Input: part model. Units: mm. Frame: model coordinates. Face numbers are marked on the shaded views. A direction names the side the tool comes from. Coordinates: 2 decimals unless noted, no trailing zeros. Write each loop counter-clockwise with the first axis right and the second up, starting at its lowest first coordinate (ties: lowest second). Pieces come first, ordered by that corner, then holes.
from build123d import *

# Parameters (mm, degrees)
SKETCH1_W            = 31.75
SKETCH1_H            = 44.45
BOSS_EXTRUDE1_DEPTH  = 4.7625
SKETCH2_R            = 1.5
SKETCH2_R_2          = 2
CUT_EXTRUDE1_DEPTH   = 5.7625
FILLET1_R            = 2.54
SKETCH3_W            = 27
SKETCH3_H            = 8
CUT_EXTRUDE2_DEPTH   = 5.7625
FILLET2_R            = 1
SKETCH4_R            = 7.9375
SKETCH4_R_2          = 4
BOSS_EXTRUDE2_DEPTH  = 4.7625
SKETCH5_R            = 4
CUT_EXTRUDE3_DEPTH   = 4.7625
SKETCH6_R            = 5.715
CUT_EXTRUDE4_DEPTH   = 3.175
CUT_REVOLVE1_ANGLE   = 90
FILLET3_R            = 5.08
FILLET3_OF_MIRROR1_R = 5.08
BOSS_EXTRUDE3_DEPTH  = 4.7625


with BuildPart() as part:
    # Sketch1 → Boss-Extrude1 (new body)
    with BuildSketch(Plane.XY):
        Rectangle(SKETCH1_W, SKETCH1_H)
    extrude(amount=BOSS_EXTRUDE1_DEPTH)

    # Sketch2 → Cut-Extrude1 (cut, through all)
    with BuildSketch(Plane.XY.offset(4.7625)):
        with Locations((-12.7, 19.05)):
            Circle(SKETCH2_R)
        with Locations((12.7, 19.05)):
            Circle(SKETCH2_R)
        with Locations((0, -17.78)):
            Circle(SKETCH2_R_2)
        with Locations((12.7, -19.05)):
            Circle(SKETCH2_R)
        with Locations((-12.7, -19.05)):
            Circle(SKETCH2_R)
    extrude(amount=-CUT_EXTRUDE1_DEPTH, mode=Mode.SUBTRACT)

    # Fillet1
    fillet1_edges = [part.edges().sort_by_distance(p)[0] for p in [
        (15.875, -22.225, 2.38125),
        (-15.875, -22.225, 2.38125),
        (-15.875, 22.225, 2.38125),
        (15.875, 22.225, 2.38125),
    ]]
    fillet(fillet1_edges, radius=FILLET1_R)

    # Sketch3 → Cut-Extrude2 (cut, through all)
    with BuildSketch(Plane.XY.offset(4.7625)):
        with Locations((0, -1.27)):
            Rectangle(SKETCH3_W, SKETCH3_H)
    extrude(amount=-CUT_EXTRUDE2_DEPTH, mode=Mode.SUBTRACT)

    # Fillet2
    fillet2_edges = [part.edges().sort_by_distance(p)[0] for p in [
        (13.5, 2.73, 2.38125),
        (13.5, -5.27, 2.38125),
        (-13.5, -5.27, 2.38125),
        (-13.5, 2.73, 2.38125),
    ]]
    fillet(fillet2_edges, radius=FILLET2_R)

    # Sketch4 → Boss-Extrude2 (add)
    with BuildSketch(Plane.XZ.offset(-2.73)):
        with Locations((0, 7.9375)):
            Circle(SKETCH4_R)
        with Locations((0, 7.9375)):
            Circle(SKETCH4_R_2, mode=Mode.SUBTRACT)
    boss_extrude2 = extrude(amount=-BOSS_EXTRUDE2_DEPTH)

    # Sketch5 → Cut-Extrude3 (cut)
    with BuildSketch(Plane.XZ.offset(-2.73)):
        with Locations((0, 7.9375)):
            Circle(SKETCH5_R)
    cut_extrude3 = extrude(amount=-CUT_EXTRUDE3_DEPTH, mode=Mode.SUBTRACT)

    # Sketch6 → Cut-Extrude4 (cut)
    with BuildSketch(Plane.XZ.offset(-7.4925)):
        with Locations((0, 7.9375)):
            Circle(SKETCH6_R)
    cut_extrude4 = extrude(amount=-CUT_EXTRUDE4_DEPTH, mode=Mode.SUBTRACT)

    # Sketch7 → Cut-Revolve1 (revolve, cut)
    with BuildSketch(Plane.XZ.offset(-10.6675)):
        with BuildLine():
            Line((5.715, 7.9375), (-5.715, 7.9375))
            ThreePointArc((-5.715, 7.9375), (0, 2.2225), (5.715, 7.9375))
        make_face()
    revolve(axis=Axis((5.715, 10.6675, 7.9375), (1, 0, 0)), revolution_arc=CUT_REVOLVE1_ANGLE, mode=Mode.SUBTRACT)

    # Fillet3
    fillet3_edges = [part.edges().sort_by_distance(p)[0] for p in [
        (7.274838916, 5.11125, 4.7625),
        (-7.274838916, 5.11125, 4.7625),
    ]]
    fillet(fillet3_edges, radius=FILLET3_R)

    # Mirror1: Boss-Extrude2, Cut-Extrude3, Cut-Extrude4 across plane
    add(boss_extrude2.mirror(Plane(origin=(0, -1.27, 0), x_dir=(0, 0, 1), z_dir=(0, -1, 0))))
    add(cut_extrude3.mirror(Plane(origin=(0, -1.27, 0), x_dir=(0, 0, 1), z_dir=(0, -1, 0))), mode=Mode.SUBTRACT)
    add(cut_extrude4.mirror(Plane(origin=(0, -1.27, 0), x_dir=(0, 0, 1), z_dir=(0, -1, 0))), mode=Mode.SUBTRACT)

    # Fillet3 of Mirror1
    fillet3_of_mirror1_edges = [part.edges().sort_by_distance(p)[0] for p in [
        (7.274838916, -7.65125, 4.7625),
        (-7.274838916, -7.65125, 4.7625),
    ]]
    fillet(fillet3_of_mirror1_edges, radius=FILLET3_OF_MIRROR1_R)

    # Sketch9 → Boss-Extrude3 (add)
    with BuildSketch(Plane.XY.offset(4.7625)):
        Polygon((-15.875, 7.4925), (-19.85, 0.897185125), (-19.85, -3.437185125), (-15.875, -10.0325), align=None)
    boss_extrude3 = extrude(amount=-BOSS_EXTRUDE3_DEPTH)

    # Mirror2: Boss-Extrude3 across plane
    add(boss_extrude3.mirror(Plane(origin=(0, 0, 0), x_dir=(0, 0, 1), z_dir=(1, 0, 0))))


solid = part.part
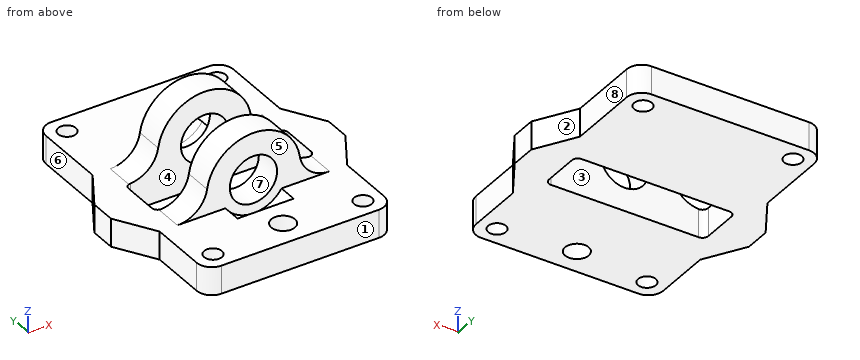
Item 1: Section query A-A, the plane y = -1. Return loops of the section in (x, z).
Item 2: Section query B-B, the plane z = 1. State how many separate pieces and enclosed holes the cut face has, then the cut area to 3 significant figures.
Item 3: Section query C-C, the plane y = 19.05. Return loops of the section in (x, z) (1 decimal).
Item 4: Pin query (flat end, axial travel): pin 1 Ø3.5 at (x, y) = (-12.7, -19.05) entering from +Z; pin 2 Ø1 at (y, z) = (7.5, 12) entering from +X; pin 3 Ø5 at (x, y) = (7, -10.5) entering from -Z; pin 4 Ø5 at (x, z) = (-9, 10.5) entering from -Y. Return the tip coordinate at first contact, or that it passes through.
Item 5: Material intervals for line 1 (Z direction, x = 0, y = -7) (1 decimal); line 2 (Y direction, x = -5, z = 6.75); line 3 (Y direction, x = 5, z = 3.25) (3 decimals), sorted ascending.
Item 6: Access query for the marked faces 4, 5, 6, 7 and 8. Directions: +Z, -Z, +X, -X, +Y, -Y. A direction counts if a zero-diameter tool reaches every point of the face in a straight line with its end or side. Return the directions, or none.
Item 7: Pull-direction query (X, two-part tool) for the marked faces 1, 2 and 3; classes: released by +X, released by -X, zero draft, split by the parting line, or undercut.
The answers:
1. outline: (-19.85, 0) - (-13.5, 0) - (-13.5, 4.76) - (-19.85, 4.76) - close; (13.5, 0) - (19.85, 0) - (19.85, 4.76) - (13.5, 4.76) - close
2. separate pieces: 1
2. enclosed holes: 6
2. area: 1,240 mm2
3. outline: (-15.9, 0) - (-14.2, 0) - (-14.2, 4.8) - (-15.9, 4.8) - close; (-11.2, 0) - (11.2, 0) - (11.2, 4.8) - (-11.2, 4.8) - close; (14.2, 0) - (15.9, 0) - (15.9, 4.8) - (14.2, 4.8) - close
4. pin 1: stops at z = 4.76
4. pin 2: stops at x = 7.09
4. pin 3: stops at z = 0
4. pin 4: stops at y = -10.03
5. line 1: z = 0 to 3.9, 11.9 to 15.9
5. line 2: y = -10.03 to -5.27, 2.73 to 7.49
5. line 3: y = -22.225 to -5.27, 2.73 to 22.225
6. face 4: +Z, -Z
6. face 5: +Z
6. face 6: +Z, -Z, -X, +Y
6. face 7: none
6. face 8: +Z, -Z, +X, +Y
7. face 1: zero draft
7. face 2: released by +X
7. face 3: undercut
